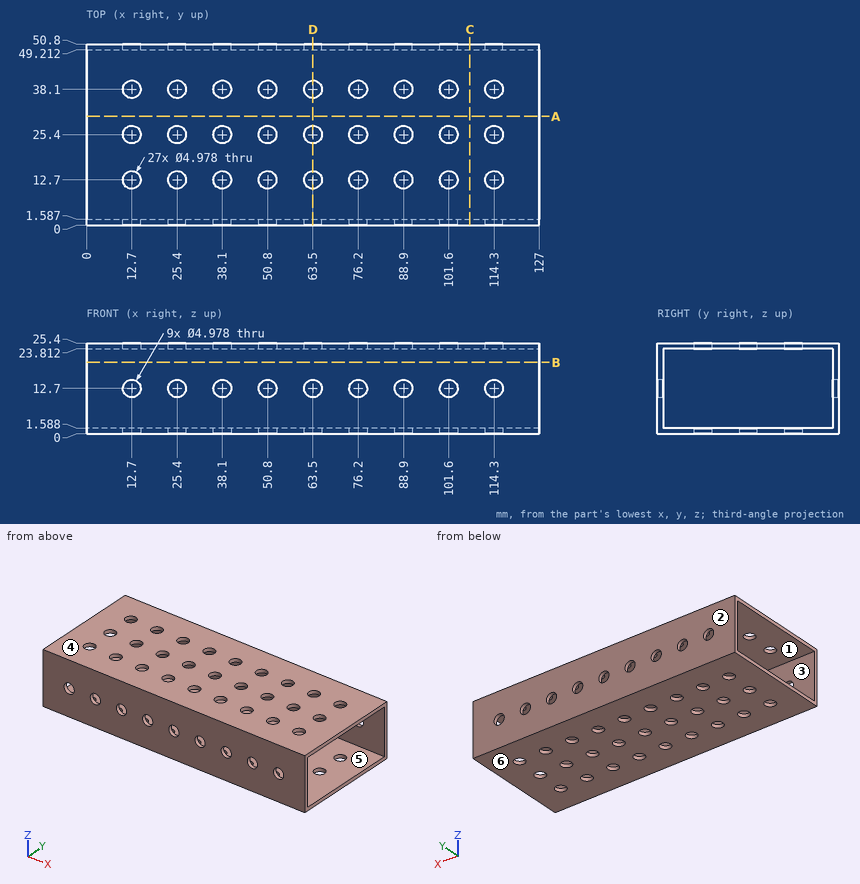
Here's the drawing with two shaded views (mm, measured from the low corner). I have some questions. A direction names the side the tool comes from. Give positions to 0.01 mm unless a question says otherwise; leave off trailing zeros. Write each loop counter-clockwise with the first axis right and the second up, starting at its lowest first coordinate (ties: lowest second). Pieces come first, ordered by that corner, then holes. Notation, with made-up numbers: (-30, 80) -> (25, 80) arc R29 ccw to (25, 104) -> close; hole circle Ø3 at (-39.75, 33). An arc over 180 degrees is marked (long way). Use one line per item in the form item = value. Start each with the question number.
1. Imagine slicing it at B-B on z = 20. List the corners of the cut face in (x, y) for me.
2. On a 3-axis mill with a long thin cutter (end or side, diameter ignored), from which of +Z, -Z, +X, -X, +Y, -Y can I reach the whole of each face in a straight line? I mean the marked faces 1 and 2. Say none if no direction works.
3. Imagine slicing it at D-D on x = 63.5. State how many separate pieces and enclosed holes the cut face has.
4. If I drill on L1, parallel to Y at x = 101.6, z = 24.65; L2, parallel to Y at x = 107.5, z = 21; L3, parallel to Z at x = 92.5, y = 26.5, over which ranges is the centre line in solid material (lowest first)?
5. Imagine slicing it at C-C on x = 107.5. List the corners of the cut face in (y, z) for me.
6. Imagine slicing it at A-A on y = 30.5. List the corners of the cut face in (x, z) for me.
7. Thinking about a two-plate mould opening in Z: for the marked faces 3, 4, 5 and 6, which applies, +Z half, -Z half, draft (parallel to the pull), parting line (faces both ways), or undercut?
Entries:
q1.outline = (0, 0) -> (127, 0) -> (127, 1.59) -> (0, 1.59) -> close; (0, 49.21) -> (127, 49.21) -> (127, 50.8) -> (0, 50.8) -> close
q2.face_1 = +X, -X
q2.face_2 = +Z, -Z, +X, -X, +Y
q3.separate_pieces = 8
q3.enclosed_holes = 0
q4.L1 = 0 to 10.21, 15.19 to 22.91, 27.89 to 35.61, 40.59 to 50.8
q4.L2 = 0 to 1.59, 49.21 to 50.8
q4.L3 = 0 to 1.59, 23.81 to 25.4
q5.outline = (0, 0) -> (50.8, 0) -> (50.8, 25.4) -> (0, 25.4) -> close; hole (1.59, 1.59) -> (49.21, 1.59) -> (49.21, 23.81) -> (1.59, 23.81) -> close
q6.outline = (0, 0) -> (127, 0) -> (127, 1.59) -> (0, 1.59) -> close; (0, 23.81) -> (127, 23.81) -> (127, 25.4) -> (0, 25.4) -> close
q7.face_3 = undercut
q7.face_4 = +Z half
q7.face_5 = undercut
q7.face_6 = -Z half
